Part model, mm, in its own coordinate system. A direction names the side the tool comes from. Coordinates: 2 decimals unless noted, no trailing zeros. Loops run counter-clockwise (first coordinate to the right, second up) from the corner with the lowest first, then second, coordinate; pieces in that order, holes last. Notation, with made-up numbers: M -10,78.25 L 22,78.25 A8 ccw 22,89.25 Z; hole C -18.5,76 d1. An arc over 180 degrees is marked long. Answer as a JSON object with one key per item and string values. Group by question number.
1. 3-axis set-ups, long thin cutter, end or side, ignore diameter. For faces 4 (the face through (-29.84, -62.61, -29.94)), 5 (the face through (0, -63, 38.1)): which of +Z, -Z, +X, -X, +Y, -Y reach the whole face in a straight line?
2. Saw through at C-C on x = 17.5. Write the cut outline in (y, z), then the cut area to 3 significant figures.
3. Saw through at B-B on z = -13. Write the cut outline in (x, y), then the cut area to 3 significant figures.
4. Drill centre lines: L1, parallel to Z at x = 5.5, y = -51.5; L2, parallel to X at y = -50.5, z = 29.5. Where is each one in solid material? Low to high.
5. Mould opens along X. For faces 1 (the face through (-36.19, -62.61, 36.29)), 2 (the face through (0, -63, -38.1)), 3 (the face through (-31.75, -63, 0)) say: released by +X, released by -X, zero draft, split by the parting line, or undercut.
6. Saw through at A-A on y = -47. Write the cut outline in (x, z).
from build123d import *

# Parameters (mm, degrees)
F1_DEPTH = 127


with BuildPart() as f1:
    # F0 (on Front) → F1 (new body)
    with BuildSketch(Plane.XZ):
        with BuildLine():
            ThreePointArc((38.1, 31.75), (36.240128, 36.240128), (31.75, 38.1))
            Line((31.75, 38.1), (-31.75, 38.1))
            ThreePointArc((-31.75, 38.1), (-36.240128, 36.240128), (-38.1, 31.75))
            Line((-38.1, 31.75), (-38.1, -31.75))
            ThreePointArc((-38.1, -31.75), (-36.240128, -36.240128), (-31.75, -38.1))
            Line((-31.75, -38.1), (31.75, -38.1))
            ThreePointArc((31.75, -38.1), (36.240128, -36.240128), (38.1, -31.75))
            Line((38.1, -31.75), (38.1, 31.75))
        make_face()
        with BuildLine():
            Line((-31.75, -25.4), (-31.75, 25.4))
            ThreePointArc((-31.75, 25.4), (-29.890128, 29.890128), (-25.4, 31.75))
            Line((-25.4, 31.75), (25.4, 31.75))
            ThreePointArc((25.4, 31.75), (29.890128, 29.890128), (31.75, 25.4))
            Line((31.75, 25.4), (31.75, -25.4))
            ThreePointArc((31.75, -25.4), (29.890128, -29.890128), (25.4, -31.75))
            Line((25.4, -31.75), (-25.4, -31.75))
            ThreePointArc((-25.4, -31.75), (-29.890128, -29.890128), (-31.75, -25.4))
        make_face(mode=Mode.SUBTRACT)
    extrude(amount=F1_DEPTH)


solid = f1.part
Outcome:
{
 "1": {"face 4": "+Y, -Y", "face 5": "+Z, +X, -X, +Y, -Y"},
 "2": {"outline": "M -127,-38.1 L 0,-38.1 L 0,-31.75 L -127,-31.75 Z; M -127,31.75 L 0,31.75 L 0,38.1 L -127,38.1 Z", "area": "1,610 mm²"},
 "3": {"outline": "M -38.1,-127 L -31.75,-127 L -31.75,0 L -38.1,0 Z; M 31.75,-127 L 38.1,-127 L 38.1,0 L 31.75,0 Z", "area": "1,610 mm²"},
 "4": {"L1": "z = -38.1 to -31.75, 31.75 to 38.1", "L2": "x = -38.1 to -30.25, 30.25 to 38.1"},
 "5": {"face 1": "released by -X", "face 2": "zero draft", "face 3": "undercut"},
 "6": {"outline": "M -38.1,-31.75 A6.35 ccw -31.75,-38.1 L 31.75,-38.1 A6.35 ccw 38.1,-31.75 L 38.1,31.75 A6.35 ccw 31.75,38.1 L -31.75,38.1 A6.35 ccw -38.1,31.75 Z; hole M -31.75,-25.4 A6.35 ccw -25.4,-31.75 L 25.4,-31.75 A6.35 ccw 31.75,-25.4 L 31.75,25.4 A6.35 ccw 25.4,31.75 L -25.4,31.75 A6.35 ccw -31.75,25.4 Z"}
}
